```python
from build123d import *

# Parameters (mm, degrees)
SKETCH1_W           = 31.75
SKETCH1_H           = 31.75
BOSS_EXTRUDE1_DEPTH = 2.54
BOSS_EXTRUDE2_DEPTH = 31.75
CUT_EXTRUDE1_DEPTH  = 42.009788671


with BuildPart() as part:
    # Sketch1 → Boss-Extrude1 (new body)
    with BuildSketch(Plane(origin=(0, 0, 0), x_dir=(1, 0, 0), z_dir=(0, 1, 0))):
        Rectangle(SKETCH1_W, SKETCH1_H)
    extrude(amount=BOSS_EXTRUDE1_DEPTH)

    # Sketch2 → Boss-Extrude2 (add, through all)
    with BuildSketch(Plane.XY.offset(15.875)):
        with BuildLine():
            ThreePointArc((10.757698592, 11.42851198), (15.254678119, 7.83956856), (13.014608296, 2.54))
            Line((13.014608296, 2.54), (15.875, 2.54))
            ThreePointArc((15.875, 2.54), (16.673544098, 9.502227526), (10.805315687, 13.332916772))
            Line((10.805315687, 13.332916772), (-14.594684313, 13.9680098))
            ThreePointArc((-14.594684313, 13.9680098), (-21.844382089, 7.62745208), (-15.875, 0.069193847))
            Line((-15.875, 0.069193847), (-15.875, 2.028572795))
            ThreePointArc((-15.875, 2.028572795), (-19.803445065, 7.604369283), (-14.642301408, 12.063605008))
            Line((-14.642301408, 12.063605008), (10.757698592, 11.42851198))
        make_face()
        with BuildLine():
            ThreePointArc((13.014608296, 2.54), (11.868328068, 2.066487883), (10.638655855, 1.905))
            Line((10.638655855, 1.905), (-14.761344145, 1.905))
            ThreePointArc((-14.761344145, 1.905), (-15.321589537, 1.93598771), (-15.875, 2.028572795))
            Line((-15.875, 2.028572795), (-15.875, 0.069193847))
            ThreePointArc((-15.875, 0.069193847), (-15.444137647, 0.021191286), (-15.011127782, 0))
            Line((-15.011127782, 0), (-14.761344145, 0))
            Line((-14.761344145, 0), (10.638655855, 0))
            ThreePointArc((10.638655855, 0), (13.548591422, 0.668514148), (15.875, 2.54))
            Line((15.875, 2.54), (13.014608296, 2.54))
        make_face()
    extrude(amount=-BOSS_EXTRUDE2_DEPTH)

    # Sketch3 → Cut-Extrude1 (cut, through all)
    with BuildSketch(Plane.XY.offset(15.875)):
        with BuildLine():
            Line((13.014608296, 2.54), (-15.875, 2.54))
            Line((-15.875, 2.54), (-15.875, 2.028572795))
            ThreePointArc((-15.875, 2.028572795), (-15.321589537, 1.93598771), (-14.761344145, 1.905))
            Line((-14.761344145, 1.905), (10.638655855, 1.905))
            ThreePointArc((10.638655855, 1.905), (11.868328068, 2.066487883), (13.014608296, 2.54))
        make_face()
        with BuildLine():
            Line((15.875, 0), (15.875, 2.54))
            ThreePointArc((15.875, 2.54), (13.548591422, 0.668514148), (10.638655855, 0))
            Line((10.638655855, 0), (15.875, 0))
        make_face()
        with BuildLine():
            Line((-15.875, 0), (-15.011127782, 0))
            ThreePointArc((-15.011127782, 0), (-15.444137647, 0.021191286), (-15.875, 0.069193847))
            Line((-15.875, 0.069193847), (-15.875, 0))
        make_face()
    extrude(amount=-CUT_EXTRUDE1_DEPTH, mode=Mode.SUBTRACT)


solid = part.part
```
Can you work these out from the model? Positions are in its coordinate system, mm. Round coordinates to 2 decimals unless told otherwise and drop trailing zeros. Order: outer loops, then holes, each group sorted by start corner. A loop starts at its lowest first (then second) coordinate and runs counter-clockwise, first axis right, second up.
(1) We'd pull the mould along X, two halves only. Please class faces 1 (the face through (-2, 1.905, 0)), 2 (the face through (-1, 1, 15.875)): +X half, -X half, draft (parallel to the pull), parting line (faces both ways), or undercut.
Results are:
face 1: undercut
face 2: draft
(2) I'm going to push flat-ended pins straight in: pin 1 (1 mm diameter, centred on x = -13, z = 4.5, fed in from +Y); pin 2 (4 mm diameter, centred on y = 7.5, z = 4.5, fed in from -X); pin 3 (6 mm diameter, centred on x = 12.5, z = -9.5, fed in from +Y); pin 4 (2 mm diameter, centred on y = 4.5, z = 4.5, fed in from +X). Where does each tip first touch, or does it pass through?
Results are:
pin 1: stops at y = 13.94
pin 2: stops at x = -21.87
pin 3: stops at y = 13.37
pin 4: stops at x = 17.2
(3) If I drill on L1, parallel to Y at x = 8, z = 6 (3 decimals); L2, parallel to Y at x = -9, z = 6 (3 decimals); L3, parallel to X at y = 10.25, z = 10.5, over which ranges is the centre line in solid material (lowest first)?
Results are:
L1: y = 0 to 1.905, 11.497 to 13.403
L2: y = 0 to 1.905, 11.923 to 13.828
L3: x = -21.06 to -18.65, 13.78 to 16.26
(4) If we section it at B-B (z = 6): Please give me the cut outline in (x, y) (1 decimal).
Results are:
outline: (-15, 0) - (10.6, 0) arc R6.7 ccw to (10.8, 13.3) - (-14.6, 14) arc R7 ccw (long way) to start; hole (-14.8, 1.9) - (10.6, 1.9) arc R4.8 ccw to (10.8, 11.4) - (-14.6, 12.1) arc R5.1 ccw (long way) to start
(5) If we section it at C-C (y = 4): Please give me the cut outline in (x, z) (3 decimals), plus the area to 3 significant figures.
Results are:
outline: (-21.203, -15.875) - (-18.872, -15.875) - (-18.872, 15.875) - (-21.203, 15.875) - close; (14.584, -15.875) - (16.749, -15.875) - (16.749, 15.875) - (14.584, 15.875) - close
area: 143 mm2
(6) If we section it at A-A (x = 8.5): Please give me the cut outline in (y, z) (3 decimals).
Results are:
outline: (0, -15.875) - (1.905, -15.875) - (1.905, 15.875) - (0, 15.875) - close; (11.485, -15.875) - (13.391, -15.875) - (13.391, 15.875) - (11.485, 15.875) - close
(7) If we section it at D-D (y = 1.25): Please give me the cut outline in (x, z) (3 decimals), plus the area to 3 significant figures.
Results are:
outline: (-18.876, -15.875) - (14.525, -15.875) - (14.525, 15.875) - (-18.876, 15.875) - close
area: 1,060 mm2
